Verification items for the finished model (mm, model axes). A direction names the side the tool comes from. Coordinates: 2 decimals unless noted, no trailing zeros. Write each loop counter-clockwise with the first axis right and the second up, starting at its lowest first coordinate (ties: lowest second). Pieces come first, ordered by that corner, then holes. Notation, with made-up numbers: (54, 71.25) -> (80, 71.25) arc R36 cw to (80, 108.25) -> close; hole circle Ø8 at (-37, 61). An arc over 180 degrees is marked (long way). Answer in a Markdown table with one row per item.
```python
from build123d import *

# Parameters (mm, degrees)
SKETCH1_W                  = 35.56
SKETCH1_H                  = 2.54
BOSS_EXTRUDE1_DEPTH        = 8.5
SKETCH2_W                  = 1
SKETCH2_H                  = 1
CUT_EXTRUDE1_DEPTH         = 8
CHAMFER1_SIZE              = 0.25
LPATTERN2_COUNT            = 14
LPATTERN2_PITCH            = 2.54
CHAMFER1_OF_LPATTERN2_SIZE = 0.25
SKETCH3_R                  = 0.5
BOSS_EXTRUDE2_DEPTH        = 3
LPATTERN3_COUNT            = 14
LPATTERN3_PITCH            = 2.54


with BuildPart() as part:
    # Sketch1 → Boss-Extrude1 (new body)
    with BuildSketch(Plane.XY):
        with Locations((17.78, 1.27)):
            Rectangle(SKETCH1_W, SKETCH1_H)
    extrude(amount=BOSS_EXTRUDE1_DEPTH)

    # Sketch2 → Cut-Extrude1 (cut)
    with BuildSketch(Plane.XY.offset(8.5)):
        with Locations((1.27, 1.27)):
            Rectangle(SKETCH2_W, SKETCH2_H)
    cut_extrude1 = extrude(amount=-CUT_EXTRUDE1_DEPTH, mode=Mode.SUBTRACT)

    # Chamfer1
    chamfer1_edges = [part.edges().sort_by_distance(p)[0] for p in [
        (0.77, 1.27, 8.5),
        (1.27, 0.77, 8.5),
        (1.77, 1.27, 8.5),
        (1.27, 1.77, 8.5),
    ]]
    chamfer(chamfer1_edges, length=CHAMFER1_SIZE)

    # LPattern2: Cut-Extrude1 ×14
    with Locations(*[(i * LPATTERN2_PITCH, 0, 0) for i in range(1, LPATTERN2_COUNT)]):
        add(cut_extrude1, mode=Mode.SUBTRACT)

    # Chamfer1 of LPattern2
    chamfer1_of_lpattern2_edges = [part.edges().sort_by_distance(p)[0] for p in [
        (3.31, 1.27, 8.5),
        (3.81, 0.77, 8.5),
        (4.31, 1.27, 8.5),
        (3.81, 1.77, 8.5),
        (5.85, 1.27, 8.5),
        (6.35, 0.77, 8.5),
        (6.85, 1.27, 8.5),
        (6.35, 1.77, 8.5),
        (8.39, 1.27, 8.5),
        (8.89, 0.77, 8.5),
        (9.39, 1.27, 8.5),
        (8.89, 1.77, 8.5),
        (10.93, 1.27, 8.5),
        (11.43, 0.77, 8.5),
        (11.93, 1.27, 8.5),
        (11.43, 1.77, 8.5),
        (13.47, 1.27, 8.5),
        (13.97, 0.77, 8.5),
        (14.47, 1.27, 8.5),
        (13.97, 1.77, 8.5),
        (16.01, 1.27, 8.5),
        (16.51, 0.77, 8.5),
        (17.01, 1.27, 8.5),
        (16.51, 1.77, 8.5),
        (18.55, 1.27, 8.5),
        (19.05, 0.77, 8.5),
        (19.55, 1.27, 8.5),
        (19.05, 1.77, 8.5),
        (21.09, 1.27, 8.5),
        (21.59, 0.77, 8.5),
        (22.09, 1.27, 8.5),
        (21.59, 1.77, 8.5),
        (23.63, 1.27, 8.5),
        (24.13, 0.77, 8.5),
        (24.63, 1.27, 8.5),
        (24.13, 1.77, 8.5),
        (26.17, 1.27, 8.5),
        (26.67, 0.77, 8.5),
        (27.17, 1.27, 8.5),
        (26.67, 1.77, 8.5),
        (28.71, 1.27, 8.5),
        (29.21, 0.77, 8.5),
        (29.71, 1.27, 8.5),
        (29.21, 1.77, 8.5),
        (31.25, 1.27, 8.5),
        (31.75, 0.77, 8.5),
        (32.25, 1.27, 8.5),
        (31.75, 1.77, 8.5),
        (33.79, 1.27, 8.5),
        (34.29, 0.77, 8.5),
        (34.79, 1.27, 8.5),
        (34.29, 1.77, 8.5),
    ]]
    chamfer(chamfer1_of_lpattern2_edges, length=CHAMFER1_OF_LPATTERN2_SIZE)

    # Sketch3 → Boss-Extrude2 (add)
    with BuildSketch(Plane(origin=(0, 0, 0), x_dir=(-1, 0, 0), z_dir=(0, 0, -1))):
        with Locations((-1.27, 1.27)):
            Circle(SKETCH3_R)
    boss_extrude2 = extrude(amount=BOSS_EXTRUDE2_DEPTH)

    # LPattern3: Boss-Extrude2 ×14
    with Locations(*[(i * LPATTERN3_PITCH, 0, 0) for i in range(1, LPATTERN3_COUNT)]):
        add(boss_extrude2)


solid = part.part
```
1. Thickness scan on line 1 (Y direction, x = 24.5, z = 5); line 2 (Z direction, x = 20.5, y = 0.95); line 3 (Z direction, x = 21, y = 1). Record the ranges inside material, lowest first. Write a range as from..to.
Geometry says:
| item | result |
|---|---|
| line 1 | 0..0.77, 1.77..2.54 |
| line 2 | 0..8.5 |
| line 3 | 0..8.34 |
2. Section check A-A, the plane z = -1. State how many separate pieces and enclosed holes the cut face has, plus the area to 3 significant figures.
Geometry says:
| item | result |
|---|---|
| separate pieces | 14 |
| enclosed holes | 0 |
| area | 11.0 mm^2 |
3. Section check B-B, the plane x = 6.35. Record the boundary of the cut face in (y, z).
Geometry says:
| item | result |
|---|---|
| outline | (0, 0) -> (0.77, 0) -> (0.77, -3) -> (1.77, -3) -> (1.77, 0) -> (2.54, 0) -> (2.54, 8.5) -> (2.02, 8.5) -> (1.77, 8.25) -> (1.77, 0.5) -> (0.77, 0.5) -> (0.77, 8.25) -> (0.52, 8.5) -> (0, 8.5) -> close |
4. Mould release check, pull along Y, two halves, no side actions. Record for faces 4 (the flat face through (29, 1, 0.5)), 5 (the cylindrical face through (16.033, 1.42, -1.479)), 6 (the flat face through (21.6, 1.3, -3)): released by +Y, released by -Y, zero draft, split by the parting line, or undercut.
Geometry says:
| item | result |
|---|---|
| face 4 | undercut |
| face 5 | split by the parting line |
| face 6 | zero draft |
5. Tool access check on faces 1 (the flat face through (11.4, 1.3, -3)), 2 (the cylindrical face through (10.953, 1.42, -1.479)), 3 (the flat face through (5.85, 1, 4)). Record the directions out of +Z, -Z, +X, -X, +Y, -Y that give a thin tool (end or side, any length) a straight path to the whole face; none if there is none.
Geometry says:
| item | result |
|---|---|
| face 1 | -Z, +X, -X, +Y, -Y |
| face 2 | -Z |
| face 3 | +Z |
6. Depth check by flat-ended pin: P1, Ø0.5, axis at y = 1.5, z = 5.5, coming from the -X side; P2, Ø0.8, axis at x = 26.5, y = 1, coming from the +Z side. Enter the tip coordinate at first touch or a pass-through.
Geometry says:
| item | result |
|---|---|
| P1 | x = 0 |
| P2 | z = 8.42 |
